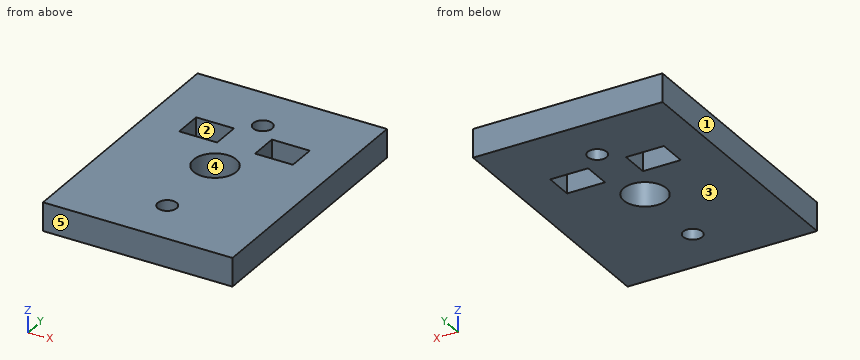
from build123d import *

# Parameters (mm, degrees)
CROQUIS1_W              = 20
CROQUIS1_H              = 27.5
CROQUIS1_R              = 2.25
CROQUIS1_R_2            = 1
CROQUIS1_W_2            = 4
CROQUIS1_H_2            = 3
SALIENTE_EXTRUIR1_DEPTH = 3


with BuildPart() as part:
    # Croquis1 → Saliente-Extruir1 (new body)
    with BuildSketch(Plane.XY):
        Rectangle(CROQUIS1_W, CROQUIS1_H)
        Circle(CROQUIS1_R, mode=Mode.SUBTRACT)
        with Locations((0, 8.5)):
            Circle(CROQUIS1_R_2, mode=Mode.SUBTRACT)
        with Locations((0, -8.5)):
            Circle(CROQUIS1_R_2, mode=Mode.SUBTRACT)
        with Locations((4, 5.25)):
            Rectangle(CROQUIS1_W_2, CROQUIS1_H_2, mode=Mode.SUBTRACT)
        with Locations((-4, 5.25)):
            Rectangle(CROQUIS1_W_2, CROQUIS1_H_2, mode=Mode.SUBTRACT)
    extrude(amount=SALIENTE_EXTRUIR1_DEPTH)


solid = part.part
Source: CAD feature listing. Evaluate the final solid. Frame: model axes, mm. Face numbers are marked on the shaded views. A direction names the side the tool comes from. Coordinates: 2 decimals unless noted, no trailing zeros. Loops run counter-clockwise (first coordinate to the right, second up) from the corner with the lowest first, then second, coordinate; pieces in that order, holes last. Notation, with made-up numbers: (75.25, -22) - (130.25, -22) arc R23 cw to (130.25, 13) - close; hole circle Ø4 at (68, 30). An arc over 180 degrees is marked (long way). Return JSON: item names as keys, results as strings.
Q1. Section B-B, the plane x = -1.5. Return loops of the section in (y, z).
Results:
{"outline": "(-13.75, 0) - (-1.68, 0) - (-1.68, 3) - (-13.75, 3) - close; (1.68, 0) - (13.75, 0) - (13.75, 3) - (1.68, 3) - close"}
Q2. Access query for the marked faces 1 and 2. Directions: +Z, -Z, +X, -X, +Y, -Y. A direction counts if a zero-diameter tool reaches every point of the face in a straight line with its end or side. Return the directions, or none.
Results:
{"face 1": "+Z, -Z, -X, +Y, -Y", "face 2": "+Z, -Z"}
Q3. Section A-A, the plane y = 6.25. Return loops of the section in (x, z).
Results:
{"outline": "(-10, 0) - (-6, 0) - (-6, 3) - (-10, 3) - close; (-2, 0) - (2, 0) - (2, 3) - (-2, 3) - close; (6, 0) - (10, 0) - (10, 3) - (6, 3) - close"}
Q4. Material intervals for line 1 along Y through (x, z) = (0, 1.45); line 2 along X through (y, z) = (4.5, 1.05); line 3 along Y through (x, z) = (-2.5, 2), sorted ascending.
Results:
{"line 1": "-13.75 to -9.5, -7.5 to -2.25, 2.25 to 7.5, 9.5 to 13.75", "line 2": "-10 to -6, -2 to 2, 6 to 10", "line 3": "-13.75 to 3.75, 6.75 to 13.75"}
Q5. Section C-C, the plane z = 0.7. Return loops of the section in (x, y), plus the area to 3 significant figures.
Results:
{"outline": "(-10, -13.75) - (10, -13.75) - (10, 13.75) - (-10, 13.75) - close; hole (-6, 3.75) - (-2, 3.75) - (-2, 6.75) - (-6, 6.75) - close; hole circle Ø4.5 at (0, 0); hole circle Ø2 at (0, -8.5); hole circle Ø2 at (0, 8.5); hole (2, 3.75) - (6, 3.75) - (6, 6.75) - (2, 6.75) - close", "area": "504 mm2"}
Q6. Mould query, pull axis Y, two halves, no side actions, for the marked faces 3, 4 and 5. Classes: released by +Y, released by -Y, zero draft, split by the parting line, or undercut.
Results:
{"face 3": "zero draft", "face 4": "undercut", "face 5": "released by -Y"}
